from build123d import *

# Parameters (mm, degrees)
PAD_DEPTH            = 10
POCKET_DEPTH         = 8.4
SKETCH002_R          = 1.5
POCKET001_DEPTH      = 34.001
POCKET001_DEPTH_BACK = -8.001
SKETCH003_R          = 3
POCKET004_DEPTH      = 1.6
POCKET005_DEPTH      = 2
FILLET_R             = 1
PAD001_DEPTH         = 1.5


with BuildPart() as fillet_body:
    # Sketch → Pad (new body)
    with BuildSketch(Plane.XY):
        with BuildLine():
            ThreePointArc((-5, 15.356513), (0, -16.15), (5, 15.356513))
            Line((5, 23), (5, 15.356513))
            Line((5, 23), (13, 23))
            Line((13, 16.492423), (13, 23))
            ThreePointArc((1.5, -20.94636), (20.074315, -6.166189), (13, 16.492423))
            Line((1.5, -20.94636), (1.5, -32.000014))
            ThreePointArc((-1.5, -32.000014), (0, -33.5), (1.5, -32.000014))
            Line((-1.5, -20.94636), (-1.5, -32.000014))
            ThreePointArc((-13, 16.492423), (-20.074315, -6.166189), (-1.5, -20.94636))
            Line((-13, 16.492423), (-13, 23))
            Line((-13, 23), (-5, 23))
            Line((-5, 23), (-5, 15.356513))
        make_face()
    extrude(amount=PAD_DEPTH)

    # Sketch001 → Pocket (cut)
    with BuildSketch(Plane.XY.offset(10)):
        with BuildLine():
            ThreePointArc((-1.5, -20.94636), (0, -21), (1.5, -20.94636))
            Line((1.5, -20.94636), (1.5, -32.000014))
            ThreePointArc((-1.5, -32.000014), (0, -33.5), (1.5, -32.000014))
            Line((-1.5, -20.94636), (-1.5, -32.000014))
        make_face()
    extrude(amount=-POCKET_DEPTH, mode=Mode.SUBTRACT)

    # Sketch002 → Pocket001 (cut, two sides)
    with BuildSketch(Plane.YZ.offset(13)) as pocket001_sk:
        with Locations((18, 5)):
            Circle(SKETCH002_R)
    extrude(amount=-POCKET001_DEPTH, mode=Mode.SUBTRACT)
    extrude(pocket001_sk.sketch, amount=-POCKET001_DEPTH_BACK, mode=Mode.SUBTRACT)

    # Sketch003 → Pocket004 (cut, symmetric)
    with BuildSketch(Plane.YZ.offset(13)):
        with Locations((18, 5)):
            Circle(SKETCH003_R)
    extrude(amount=POCKET004_DEPTH, both=True, mode=Mode.SUBTRACT)

    # Sketch004 → Pocket005 (cut, symmetric)
    with BuildSketch(Plane(origin=(-13, 0, 0), x_dir=(0, -1, 0), z_dir=(-1, 0, 0))):
        Polygon((-18, 8.3), (-20.857884, 6.65), (-20.857884, 3.35), (-18, 1.7), (-15.142116, 3.35), (-15.142116, 6.65), align=None)
    extrude(amount=POCKET005_DEPTH, both=True, mode=Mode.SUBTRACT)

    # Fillet
    fillet_edges = [fillet_body.edges().sort_by_distance(p)[0] for p in [
        (-20.074315, -6.166189, 10),
        (0, -21, 10),
        (20.074315, -6.166189, 10),
        (13, 19.746211, 10),
        (9, 23, 10),
        (-9, 23, 10),
        (-13, 19.746211, 10),
    ]]
    fillet(fillet_edges, radius=FILLET_R)


with BuildPart() as fusion:
    # Sketch005 → Pad001 (new body, symmetric)
    with BuildSketch(Plane.YZ):
        with BuildLine():
            Line((-26, 1.6), (-20, 1.6))
            Line((-20, 1.6), (-20, 9.5))
            ThreePointArc((-26, 1.6), (-21.359014, 4.303682), (-20, 9.5))
        make_face()
    extrude(amount=PAD001_DEPTH, both=True)

    # Fusion: union Fillet body
    add(fillet_body.part)


solid = fusion.part
Verification items for the finished model (mm, model axes). A direction names the side the tool comes from. Coordinates: 2 decimals unless noted, no trailing zeros. Order: outer loops, then holes, each group sorted by start corner. A loop starts at its lowest first (then second) coordinate and runs counter-clockwise, first axis right, second up.
1. Sectioned sample at C-C, the plane y = -30. Record the cut outline in (x, z), and give its area (3 significant figures).
Results found:
outline: (-1.5, 0) - (1.5, 0) - (1.5, 1.6) - (-1.5, 1.6) - close
area: 4.80 mm2
2. Scan lines: line 1 (Z direction, x = 12, y = 18); line 2 (X direction, y = 0, z = 7); line 3 (Y direction, x = 9, z = 5.25). Record each from-to range of solid material in increasing order.
Results found:
line 1: z = 0 to 2, 8 to 10
line 2: x = -21 to -16.15, 16.15 to 21
line 3: y = -18.97 to -13.41, 13.41 to 16.52, 19.48 to 23
3. Go/stop test with flat-tipped pins: pin 1 Ø4 at (x, z) = (7, 4.5) entering from -Y; pin 2 Ø5 at (y, z) = (9, 8.5) entering from -X; pin 3 Ø3 at (y, z) = (0.5, 8) entering from +X; pin 4 Ø1.7 at (y, z) = (19, 3.5) entering from -X. Record where each tip stops, or that it passes through.
Results found:
pin 1: stops at y = -20.4
pin 2: stops at x = -19.97
pin 3: stops at x = 21
pin 4: stops at x = -11
4. Sectioned sample at D-D, the plane y = -23. Record the cut outline in (x, z), and give its area (3 significant figures).
Results found:
outline: (-1.5, 0) - (1.5, 0) - (1.5, 2.75) - (-1.5, 2.75) - close
area: 8.24 mm2
5. Sectioned sample at B-B, the plane x = 0. Record the cut outline in (y, z), and give its area (3 significant figures).
Results found:
outline: (-33.5, 0) - (-16.15, 0) - (-16.15, 10) - (-20, 10) arc R1 ccw to (-21, 9) - (-21, 4.82) arc R7 cw to (-26, 1.6) - (-33.5, 1.6) - close
area: 73.7 mm2
6. Release check for a two-part mould opening along Y. For faces 1 (the face through (-12.406, 16.591, 2.513)), 2 (the face through (-5, 20, 5)), 3 (the face through (19.97, -6.5, 4.44)), 4 (the face through (-13, 15.142, 5)) record: +Y half, -Y half, draft (parallel to the pull), parting line (faces both ways), or undercut.
Results found:
face 1: undercut
face 2: draft
face 3: parting line
face 4: undercut
7. Sectioned sample at A-A, the plane x = 6. Give the number of separate pieces and of enclosed holes in the cut face, and give its area (3 significant figures).
Results found:
separate pieces: 2
enclosed holes: 1
area: 124 mm2
8. Set-up check for faces 5 (the face through (-12, 20.858, 5)), 6 (the face through (0, -21, 7)), 7 (the face through (13, 21, 4)): record each of +Z, -Z, +X, -X, +Y, -Y from which the full face is reachable in a straight line by a thin tool's end or side.
Results found:
face 5: -X
face 6: +Z, -Y
face 7: +Z, -Z, +X, +Y
